from build123d import *

# Parameters (mm, degrees)
SKETCH_1_W                = 110
SKETCH_1_H                = 30
EXTRUDE_1_DEPTH           = 20
EXTRUDE_2_DEPTH           = 5
EXTRUDE_2_DEPTH_BACK      = 20
FILLET_1_R                = 1
CUT_EXTRUDE_1_DEPTH       = 20
HOLE_WIZARD_1_D           = 8
HOLE_WIZARD_1_DEPTH       = 20
HOLE_WIZARD_1_CBORE_D     = 12
HOLE_WIZARD_1_CBORE_DEPTH = 5
CUT_EXTRUDE_2_REACH       = 32
SKETCH_7_W                = 20
SKETCH_7_H                = 20


with BuildPart() as part:
    # 草图1 → 凸台-拉伸1 (new body)
    with BuildSketch(Plane.XY):
        with Locations((-5, 0)):
            Rectangle(SKETCH_1_W, SKETCH_1_H)
    extrude(amount=EXTRUDE_1_DEPTH)

    # 草图3 → 凸台-拉伸2 (add, two sides)
    with BuildSketch(Plane.XY.offset(20)) as extrude_2_sk:
        Polygon((-60, -15), (-60, 15), (-75, 15), (-85, 5), (-85, -10), (-105, -10), (-105, -15), align=None)
    extrude(amount=EXTRUDE_2_DEPTH)
    extrude(extrude_2_sk.sketch, amount=-EXTRUDE_2_DEPTH_BACK)

    # 圆角1
    fillet_1_edges = [part.edges().sort_by_distance(p)[0] for p in [
        (-60, 15, 22.5),
        (-60, 0, 25),
        (-60, 0, 20),
        (-5, 15, 20),
    ]]
    fillet(fillet_1_edges, radius=FILLET_1_R)

    # 草图4 → 切除-拉伸1 (cut)
    with BuildSketch(Plane.XZ.offset(15)):
        with BuildLine():
            Line((-94.259340252, 25), (-99.916194502, 19.343145751))
            Line((-99.916194502, 19.343145751), (-90.484708185, 13.897874587))
            Line((-90.484708185, 13.897874587), (-77.622420706, 13.897874587))
            ThreePointArc((-77.622420706, 13.897874587), (-72.004883636, 12.451966115), (-77.602894826, 10.932214568))
            Line((-77.602894826, 10.932214568), (-92.230981332, 10.932214568))
            Line((-92.230981332, 10.932214568), (-90.609831702, 7.106640556))
            ThreePointArc((-90.609831702, 7.106640556), (-91.670953588, 4.484805255), (-94.292788888, 5.545927141))
            Line((-94.292788888, 5.545927141), (-96.339745962, 10.376317651))
            Line((-96.339745962, 10.376317651), (-105, 15.376317651))
            Line((-105, 15.376317651), (-105, 25))
            Line((-105, 25), (-94.259340252, 25))
        make_face()
    extrude(amount=-CUT_EXTRUDE_1_DEPTH, mode=Mode.SUBTRACT)

    # 孔1
    with Locations(Plane(origin=(-75, -2, 25), x_dir=(1, 0, 0), z_dir=(0, 0, 1))):
        with Locations((0, 0)):
            CounterBoreHole(HOLE_WIZARD_1_D / 2, HOLE_WIZARD_1_CBORE_D / 2, HOLE_WIZARD_1_CBORE_DEPTH, depth=HOLE_WIZARD_1_DEPTH)

    # 草图7 → 切除-拉伸2 (cut, up to next)
    with BuildSketch(Plane(origin=(0, -15, 0), x_dir=(-1, 0, 0), z_dir=(0, -1, 0)), mode=Mode.PRIVATE) as cut_extrude_2_sk1:
        with Locations((-40, -10)):
            Rectangle(SKETCH_7_W, SKETCH_7_H)
    cut_extrude_2_tool1 = extrude(cut_extrude_2_sk1.sketch, amount=-CUT_EXTRUDE_2_REACH, mode=Mode.PRIVATE) & part.part
    add(cut_extrude_2_tool1.solids().sort_by_distance((40, -15, 10))[0], mode=Mode.SUBTRACT)


solid = part.part
The model under review builds one solid part; all positions refer to its coordinate system, in mm. A direction names the side the tool comes from. Round coordinates to 2 decimals unless told otherwise and drop trailing zeros. Loops run counter-clockwise (first coordinate to the right, second up) from the corner with the lowest first, then second, coordinate; pieces in that order, holes last. Notation, with made-up numbers: (1.25, 64) -> (27.25, 64) arc R28 cw to (27.25, 85) -> close; hole circle Ø2 at (78.25, -1). An arc over 180 degrees is marked (long way). Write item = value, one per line. Start each with the question number.
Item 1: Mouldability with a two-part tool opening along Z and no side actions: class faces 1 (the cylindrical face through (-91.631, -12.535, 4.502)), 2 (the flat face through (-85, -2, 6)), 3 (the flat face through (-23, 0, 0)) as released by +Z, released by -Z, zero draft, split by the parting line, or undercut.
Item 2: Take a section at A-A on y = -2. Give the boundary of the cut face in (x, z), plus the area to 3 significant figures.
Item 3: Take a section at B-B on z = 12.25. Give the boundary of the cut face in (x, y), plus the area to 3 significant figures.
Item 4: Take a section at C-C on y = 10. Give the boundary of the cut face in (x, z), plus the area to 3 significant figures.
Item 5: For faces 4 (the flat face through (-91.432, -12.535, 9.046)), 5 (the flat face through (-75, -2, 5)), 6 (the flat face through (-78, 5, 12)), 7 (the flat face through (-95, -10, 6)), 8 (the flat face through (-60, -1, 22)), list the 3-axis set-ups (+Z, -Z, +X, -X, +Y, -Y) from which the entire face can be reached by the end or side of a thin tool; tool diameter is ignored.
Item 6: Take a section at D-D on x = -41.5. Give the boundary of the cut face in (y, z).
Item 7: To check wall thickness, follow L1, parallel to Y at x = -75, z = 21.6; L2, parallel to Z at x = -82, y = -4.5; L3, parallel to X at y = -7.5, z = 18. State the ranges of each line that lie inside material, in increasing order.
Item 8: Insertion check: pin 1 (3.5 mm diameter, centred on y = -5, z = 6, fed in from -X); pin 2 (4 mm diameter, centred on y = 10, z = 16.5, fed in from -X); pin 3 (4 mm diameter, centred on x = -75, y = -1.5, fed in from +Z). Each pin has a flat end and moves straight along its axis. Give the tip position at first contact, or say it passes through.
Result:
q1.face_1 = undercut
q1.face_2 = zero draft
q1.face_3 = released by -Z
q2.outline = (-85, 0) -> (30, 0) -> (30, 20) -> (-59, 20) arc R1 cw to (-60, 21) -> (-60, 24) arc R1 ccw to (-61, 25) -> (-69, 25) -> (-69, 20) -> (-71, 20) -> (-71, 5) -> (-79, 5) -> (-79, 10.93) -> (-85, 10.93) -> close; (-85, 13.9) -> (-79, 13.9) -> (-79, 20) -> (-81, 20) -> (-81, 25) -> (-85, 25) -> close
q2.area = 2,230 mm²
q3.outline = (-105, -15) -> (-99.59, -15) -> (-99.59, -10) -> (-105, -10) -> close; (-85, 5) -> (-72.01, 5) -> (-72.01, 0.66) arc R4 cw to (-72.01, -4.66) -> (-72.01, -15) -> (30, -15) -> (30, 15) -> (-75, 15) -> close
q3.area = 3,160 mm²
q4.outline = (-80, 0) -> (30, 0) -> (30, 20) -> (-59, 20) arc R1 cw to (-60, 21) -> (-60, 24) arc R1 ccw to (-61, 25) -> (-80, 25) -> close
q4.area = 2,300 mm²
q5.face_4 = +Y, -Y
q5.face_5 = +Z
q5.face_6 = -Y
q5.face_7 = +Z, -Z, -X, +Y
q5.face_8 = +Z, +X, +Y, -Y
q6.outline = (-15, 0) -> (15, 0) -> (15, 19) arc R1 ccw to (14, 20) -> (-15, 20) -> close
q7.L1 = -15 to -8, 4 to 15
q7.L2 = 0 to 10.93, 13.9 to 25
q7.L3 = -85 to 30
q8.pin_1 = -85
q8.pin_2 = -82
q8.pin_3 = 5
